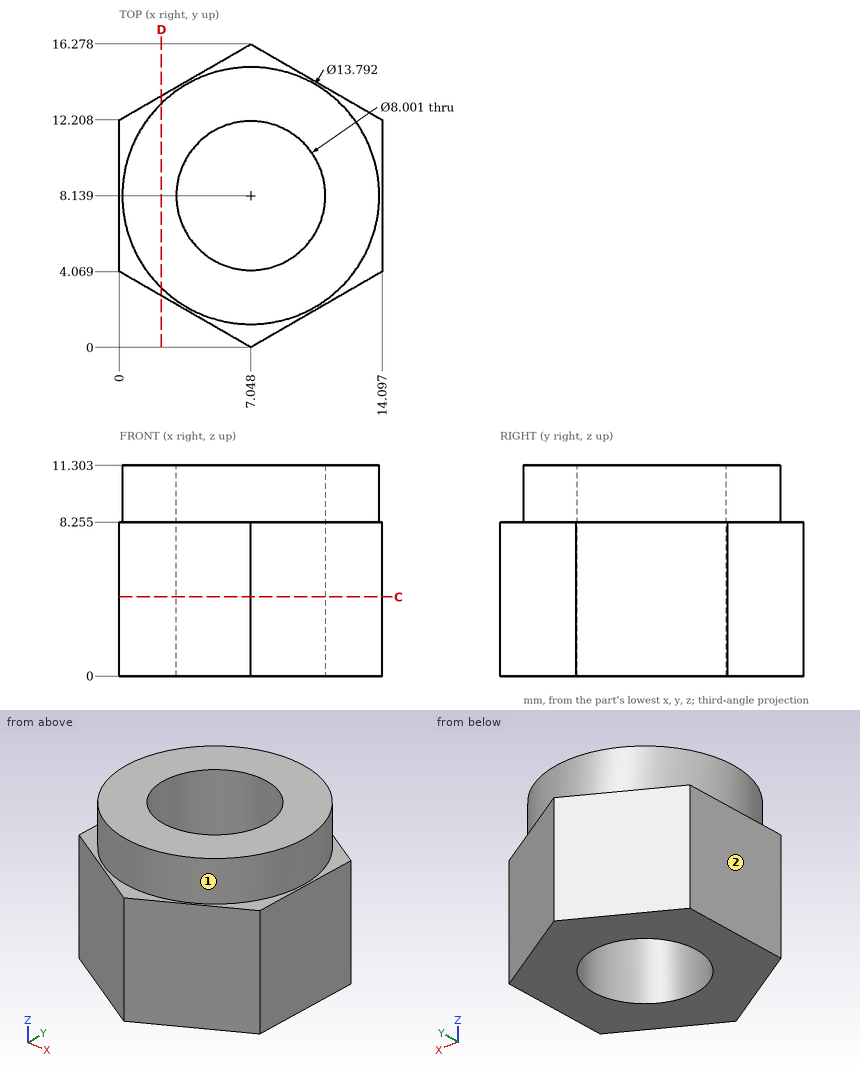
Geometry check sheet. Reference: drawing and pictorial views, mm from the part's lowest x, y, z. A direction names the side the tool comes from. Give positions to 0.01 mm unless a question says otherwise; leave off trailing zeros. Order: outer loops, then holes, each group sorted by start corner. A loop starts at its lowest first (then second) coordinate and runs counter-clockwise, first axis right, second up. Notation, with made-up numbers: M 10.5,74 L 44.5,74 A15 cw 44.5,94 Z; hole C 85.5,48 d2. An arc over 180 degrees is marked long. Answer in a Markdown table with one row per item. Add a question column.
Q1. Access from +Z, -Z, +X, -X, +Y, -Y to the whole of each face (thin tool, end or side, straight path). Record for the marked faces 1 and 2.
Q2. Thickness scan on L1, parallel to X at y = 11.25, z = 1.75 (1 decimal); L2, parallel to Y at x = 9.25, z = 1.75 (1 decimal); L3, parallel to Z at x = 13.25, y = 11.75 (1 decimal). Record the ranges inside material, lowest first.
Q3. Sectioned sample at C-C, the plane z = 4.25. Record the boundary of the cut face in (x, y), and give its area (3 significant figures).
Q4. Gauge pin test, flat ends, axial feed: pin 1 Ø1 at (y, z) = (2.5, 1.5) entering from +X (1 decimal); pin 2 Ø1 at (x, z) = (12, 6) entering from +Y; pin 3 Ø1 at (y, z) = (14.5, 4.5) entering from -X (1 decimal). Record the tip position at first contact, or that the pin passes through.
Q5. Sectioned sample at D-D, the plane x = 2.25. Record the boundary of the cut face in (y, z) (1 decimal), and give its area (3 significant figures).
Verdict:
| question | item | result |
|---|---|---|
| 1 | face 1 | +Z |
| 1 | face 2 | +Z, -Z, -X, +Y, -Y |
| 2 | L1 | 0 to 4.5, 9.6 to 14.1 |
| 2 | L2 | 1.3 to 4.8, 11.5 to 15 |
| 2 | L3 | 0 to 8.3 |
| 3 | outline | M 0,4.07 L 7.05,0 L 14.1,4.07 L 14.1,12.21 L 7.05,16.28 L 0,12.21 Z; hole C 7.05,8.14 d8 |
| 3 | area | 122 mm² |
| 4 | pin 1 | x = 12.2 |
| 4 | pin 2 | y = 13.71 |
| 4 | pin 3 | x = 3.1 |
| 5 | outline | M 2.8,0 L 13.5,0 L 13.5,8.3 L 13.1,8.3 L 13.1,11.3 L 3.2,11.3 L 3.2,8.3 L 2.8,8.3 Z |
| 5 | area | 119 mm² |
